Autodesk Inventor part; units mm, degrees
ref_plane "YZ Plane" through (0, 0, 0) normal (1, 0, 0) x (0, 1, 0)
ref_plane "XZ Plane" through (0, 0, 0) normal (0, 1, 0) x (-1, 0, 0)
ref_plane "XY Plane" through (0, 0, 0) normal (0, 0, 1) x (1, 0, 0)
sketch "Sketch1" plane through (0, 0, 0) normal (0, 0, 1) x (1, 0, 0)
  line L0 (-38.9, 0) -> (38.9, 0)
  line L1 (-38.9, 0) -> (-38.9, 2.9)
  line L2 (38.9, 0) -> (38.9, 2.9)
  line L3 (-30, 2.9) -> (-38.9, 2.9)
  line L4 (30, 2.9) -> (38.9, 2.9)
  line L5 (30, 2.9) -> (30, 27.9)
  line L6 (-30, 2.9) -> (-30, 27.9)
  line L7 (-30, 27.9) -> (30, 27.9) construction
  line L8 (-28, 41) -> (28, 41)
  line L9 (-30, 27.9) -> (-28, 41)
  line L10 (30, 27.9) -> (28, 41)
  point P0 (0, 0)
  point P1 (0, 0)
  point P2 (0, 27.9)
  point P3 (0, 41)
  dimension "d0" = 77.8
  dimension "d1" = 2.9
  dimension "d6" = 25
  dimension "d7" = 56
  dimension "d8" = 41
extrude "Extrusion1" add sketch "Sketch1" along normal blind 115
fillet "Fillet1" radius 5.75 2 edges at (28, 41, 57.5) (-28, 41, 57.5)
fillet "Fillet2" radius 20 2 edges at (-30, 27.9, 57.5) (30, 27.9, 57.5)
sketch "Sketch2" plane through (-38.9, 0, 0) normal (0, -1, 0) x (1, 0, 0)
  line L0 (0, 0) -> (77.8, 0)
  line L1 (0, 0) -> (0, 115)
  line L2 (77.8, 0) -> (77.8, 115)
  line L3 (0, 115) -> (77.8, 115)
  point P0 (38.9, 0)
  point P1 (4, 13.75)
  point P2 (73.8, 13.75)
  point P3 (4, 101)
  point P4 (73.8, 101)
  dimension "d11" = 13.75
  dimension "d12" = 4
  dimension "d13" = 4
  dimension "d14" = 14
hole "Hole1" at (-34.9, 0, 13.75) at (34.9, 0, 13.75) at (-34.9, 0, 101) at (34.9, 0, 101) direction (0, 1, 0) diameter 4.7 end through all
sketch "Sketch3" plane through (0, 0, 0) normal (0, 0, -1) x (-1, 0, 0)
  circle A0 centre (20.3461, 28.3) radius 2.425
  circle A1 centre (20.3461, 22.3) radius 2.425
  line L0 (-23.0612, 41) -> (23.0612, 41)
  point P0 (0, 0)
  dimension "d22" = 4.85
  dimension "d23" = 4.85
  dimension "d24" = 6
  dimension "d25" = 12.7
extrude "Extrusion2" add sketch "Sketch3" along normal blind 6.5
fillet "Fillet3" radius 2.25 2 edges at (-17.9211, 28.3, -6.5) (-17.9211, 22.3, -6.5)
equation "\"d23\" = d22"
properties part number "KellyController-KBS-Small"
Input: part model. Units: mm. Frame: model coordinates. A direction names the side the tool comes from. Give positions to 0.01 mm unless a question says otherwise; leave off trailing zeros. Order: outer loops, then holes, each group sorted by start corner. A loop starts at its lowest first (then second) coordinate and runs counter-clockwise, first axis right, second up. Notation, with made-up numbers: (11, -0.5) - (43, -0.5) arc R12 ccw to (43, 9.5) - close; hole circle Ø1 at (58, 89). An arc over 180 degrees is marked (long way). One line per item, written item: value.
1. Cut plane C-C, the plane z = 78. Output: boundary loops of the cut face in (x, y), and give its area (3 significant figures).
Determined:
outline: (-38.9, 0) - (38.9, 0) - (38.9, 2.9) - (30, 2.9) - (30, 26.38) arc R20 ccw to (29.77, 29.4) - (28.75, 36.12) arc R5.75 ccw to (23.06, 41) - (-23.06, 41) arc R5.75 ccw to (-28.75, 36.12) - (-29.77, 29.4) arc R20 ccw to (-30, 26.38) - (-30, 2.9) - (-38.9, 2.9) - close
area: 2,480 mm2
2. Draft query along Y for faces 1 (the face through (-29.94, 27.92, 58.3)), 2 (the face through (-18.56, 20.66, -2.1)), 3 (the face through (-35.003, 1.47, 103.348)), 4 (the face through (-1, 0, 57)). Return one class per face: released by +Y, released by -Y, zero draft, split by the parting line, or undercut.
Determined:
face 1: released by +Y
face 2: undercut
face 3: zero draft
face 4: released by -Y
3. Cut plane D-D, the plane y = 5.5. Output: boundary loops of the cut face in (x, z), and give its area (3 significant figures).
Determined:
outline: (-30, 0) - (30, 0) - (30, 115) - (-30, 115) - close
area: 6,900 mm2
4. Cut plane A-A, the plane z = 101. Output: boundary loops of the cut face in (x, y).
Determined:
outline: (-38.9, 0) - (-37.25, 0) - (-37.25, 2.9) - (-38.9, 2.9) - close; (-32.55, 0) - (32.55, 0) - (32.55, 2.9) - (30, 2.9) - (30, 26.38) arc R20 ccw to (29.77, 29.4) - (28.75, 36.12) arc R5.75 ccw to (23.06, 41) - (-23.06, 41) arc R5.75 ccw to (-28.75, 36.12) - (-29.77, 29.4) arc R20 ccw to (-30, 26.38) - (-30, 2.9) - (-32.55, 2.9) - close; (37.25, 0) - (38.9, 0) - (38.9, 2.9) - (37.25, 2.9) - close
5. Cut plane B-B, the plane x = -34.9. Output: boundary loops of the cut face in (y, z), and give its area (3 significant figures).
Determined:
outline: (0, 0) - (2.9, 0) - (2.9, 11.4) - (0, 11.4) - close; (0, 16.1) - (2.9, 16.1) - (2.9, 98.65) - (0, 98.65) - close; (0, 103.35) - (2.9, 103.35) - (2.9, 115) - (0, 115) - close
area: 306 mm2
6. Pin query (flat end, axial travel): pin 1 Ø11.5 at (y, z) = (15.5, 43.5) entering from +X; pin 2 Ø2.5 at (x, z) = (36, 54) entering from +Y; pin 3 Ø12.5 at (x, y) = (13, 29) entering from -Z. Return the tip coordinate at first contact, or that it passes through.
Determined:
pin 1: x = 30
pin 2: y = 2.9
pin 3: z = 0
7. Line query: probe 1 along Z at (x, y) = (-34.9, 1.2); probe 2 along X at (y, z) = (1.85, 101); probe 3 along Z at (x, y) = (-34, 2). Output: solid intervals per line, ascending.
Determined:
probe 1: 0 to 11.4, 16.1 to 98.65, 103.35 to 115
probe 2: -38.9 to -37.25, -32.55 to 32.55, 37.25 to 38.9
probe 3: 0 to 11.58, 15.92 to 98.83, 103.17 to 115
8. Reachability of faces 5 (the face through (-1, 21, 115)), 6 (the face through (-32.606, 1.47, 14.259)), 7 (the face through (-18.56, 26.66, -2.1)), 8 (the face through (34, 2.9, 57)), 9 (the face through (-34, 2.9, 57)) from +Z, -Z, +X, -X, +Y, -Y: full face, straight path, thin tool, end or side. Return the list, or none.
Determined:
face 5: +Z, +X, -X, +Y, -Y
face 6: +Y, -Y
face 7: -Z
face 8: +Z, -Z, +X, +Y
face 9: +Z, -Z, -X, +Y
